from build123d import *

# Parameters (mm, degrees)
F1_DEPTH = 63.5
F0_W     = 24.577054
F0_H     = 19.05
F2_DEPTH = 25.4
F3_DEPTH = 7.9375
F0_W_2   = 25.4
F0_H_2   = 28.575
F5_R     = 6.35


with BuildPart() as f1:
    # F0 (on Front) → F1 (new body, symmetric)
    with BuildSketch(Plane.XZ):
        Polygon((41.275, -9.525), (41.275, 9.525), (22.225, 9.525), (-41.275, 9.525), (-41.275, -9.525), align=None)
    extrude(amount=F1_DEPTH, both=True)

    # F0 (on Front) → F2 (join, symmetric)
    with BuildSketch(Plane.XZ):
        with BuildLine():
            Line((22.225, 9.525), (41.275, 9.525))
            Line((41.275, 9.525), (41.275, 27.0002))
            ThreePointArc((41.275, 27.0002), (45.92468, 38.22552), (57.15, 42.8752))
            Line((57.15, 42.8752), (60.325, 42.8752))
            Line((60.325, 42.8752), (60.325, 61.9252))
            Line((60.325, 61.9252), (57.15, 61.9252))
            add(Edge.make_bspline(
                [(55.929647, 61.903873), (56.335616, 61.911845), (56.742404, 61.918954), (57.15, 61.9252)],
                knots=[110.709281, 110.709281, 110.709281, 110.709281, 111.504536, 111.504536, 111.504536, 111.504536], degree=3))
            ThreePointArc((55.929647, 61.903873), (32.02654, 51.260608), (22.225, 27.0002))
            Line((22.225, 27.0002), (22.225, 9.525))
        make_face()
        with Locations((72.613527, 52.4002)):
            Rectangle(F0_W, F0_H)
    extrude(amount=F2_DEPTH, both=True)

    # F0 (on Front) → F3 (join, symmetric)
    with BuildSketch(Plane.XZ):
        with BuildLine():
            Line((-41.275, 9.525), (22.225, 9.525))
            Line((22.225, 9.525), (22.225, 27.0002))
            ThreePointArc((22.225, 27.0002), (32.02654, 51.260608), (55.929647, 61.903873))
            add(Edge.make_bspline(
                [(-41.275, 9.525), (-41.25457, 42.958838), (-0.586359, 60.794032), (55.929647, 61.903873)],
                knots=[0, 0, 0, 0, 110.709281, 110.709281, 110.709281, 110.709281], degree=3))
        make_face()
    extrude(amount=F3_DEPTH, both=True)

    # F0 (on Front) → F4 (revolve)
    with BuildSketch(Plane.XZ):
        with Locations((98.425, 52.3875)):
            Rectangle(F0_W_2, F0_H_2)
    revolve(axis=Axis((85.725, 0, 52.3875), (0, 0, 1)))

    # F5
    f5_edges = [f1.edges().sort_by_distance(p)[0] for p in [
        (-41.275, -63.5, 0),
        (41.275, -63.5, 0),
        (41.275, 63.5, 0),
        (-41.275, 63.5, 0),
    ]]
    fillet(f5_edges, radius=F5_R)


solid = f1.part
Can you work these out from the model? Positions are in its coordinate system, mm. A direction names the side the tool comes from. Round coordinates to 2 decimals unless told otherwise and drop trailing zeros. Order: outer loops, then holes, each group sorted by start corner. A loop starts at its lowest first (then second) coordinate and runs counter-clockwise, first axis right, second up. Notation, with made-up numbers: (-7.75, 65) -> (49.25, 65) arc R13 cw to (49.25, 86) -> close; hole circle Ø1 at (84, 47.5). An arc over 180 degrees is marked (long way). Write each question's results on one line, items separated by ' | '. Start each with the question number.
Item 1: Please list where these lines run through material, in increasing order: L1, parallel to Y at x = 31, z = 41.5; L2, parallel to Z at x = -24.5, y = -16 (3 decimals); L3, parallel to X at y = -14, z = 38.5.
Item 2: Which directions (+Z, -Z, +X, -X, +Y, -Y) give clear straight access to the entire face, cutting with the end or side of a thin tool? Please do faces 4 (the flat face through (60, 2, 42.875)), 5 (the flat face through (86, 0, 38.1)), 6 (the cylindrical face through (32.29, 16.55, 51.53)), 7 (the flat face through (60, 4, 61.925)), 8 (the cylindrical face through (32.29, -16.79, 51.53)).
Item 3: If we section it at B-B, the plane y = 49.5: Write out the boundary of the cut face in (x, z) (3 decimals), then the cut area to 3 significant figures.
Item 4: Thinking about a two-plate mould opening in X: for faces 1 (the cylindrical face through (45.8, -0.4, 38.1)), 2 (the flat face through (-4, 7.938, 30)), 3 (the cylindrical face through (39.464, 61.59, 0.133)), which applies, +X half, -X half, draft (parallel to the pull), parting line (faces both ways), or undercut?
Item 5: Will these pins go through, and if not, where does the flat tip stop? pin 1 (8 mm diameter, centred on y = -11, z = 48, fed in from +X); pin 2 (16.5 mm diameter, centred on x = -3.5, y = 25.5, fed in from +Z) (3 decimals); pin 3 (14 mm diameter, centred on x = 78, y = -2, fed in from -Z).
Item 6: If we section it at A-A, the plane z = 2: Write out the boundary of the cut face in (x, y) (3 decimals), then the cut area to 3 significant figures.
Results:
1) L1: y = -25.4 to 25.4 | L2: z = -9.525 to 9.525 | L3: x = 24.17 to 46.21, 64.53 to 106.92
2) face 4: -Z | face 5: -Z, +X, +Y, -Y | face 6: +Z, -X, +Y | face 7: +Z, -X | face 8: +Z, -X, -Y
3) outline: (-41.275, -9.525) -> (41.275, -9.525) -> (41.275, 9.525) -> (-41.275, 9.525) -> close | area: 1,570 mm2
4) face 1: undercut | face 2: draft | face 3: +X half
5) pin 1: stops at x = 110.14 | pin 2: stops at z = 9.525 | pin 3: stops at z = 38.1
6) outline: (-41.275, -57.15) arc R6.35 ccw to (-34.925, -63.5) -> (34.925, -63.5) arc R6.35 ccw to (41.275, -57.15) -> (41.275, 57.15) arc R6.35 ccw to (34.925, 63.5) -> (-34.925, 63.5) arc R6.35 ccw to (-41.275, 57.15) -> close | area: 10,400 mm2
